Here's how the part is built. I have some questions about the finished solid (model axes, mm). Coordinates: 2 decimals unless noted, no trailing zeros. Order: outer loops, then holes, each group sorted by start corner. A loop starts at its lowest first (then second) coordinate and runs counter-clockwise, first axis right, second up. Notation, with made-up numbers: (74, 65) - (87, 65) arc R23 ccw to (87, 98) - close; hole circle Ø4 at (22, 48.5). An arc over 180 degrees is marked (long way). Answer as CSV lines item,"result". Start each with the question number.
Item 1: Imagine slicing it at A-A on y = 546. List the corners of the cut face in (x, z) for me, and give its area (3 significant figures).
Item 2: Imagine slicing it at B-B on y = 535. List the corners of the cut face in (x, z) for me, and give its area (3 significant figures).
Item 3: I need wall thicknesses on line 1 (Y direction, x = -537, z = -80.75); line 2 (X direction, y = 515.5, z = -81); line 3 (X direction, y = 514, z = -82.75). Which ranges of each line are inside material? Lowest first, please.
Item 4: Imagine slicing it at C-C on x = -570. Count the separate pieces of the cut face and the enclosed holes in it, and give its area (3 significant figures).
Item 5: We'd pull the mould along Y, two halves only. Please class faces 1 (the face through (-650.1, 527.3, -81)), 2 (the face through (-530.587, 524, -81)), 3 (the face through (-549, 531.139, -82)), 4 (the face through (-566, 513.156, -82)): pulls with the +Y half, pulls with the -Y half, needs draft (parallel to the pull), parting line crosses it, or undercut.
Item 6: I'm going to push flat-ended pins straight in: pin 1 (3 mm diameter, centred on x = -634, z = -81, fed in from -Y); pin 2 (1.4 mm diameter, centred on y = 511.5, z = -82, fed in from -X); pin 3 (1.3 mm diameter, centred on y = 499.5, z = -79, fed in from -X); pin 4 (4 mm diameter, centred on x = -569.5, y = 534.5, fed in from -Z). Where does each tip first touch, or does it pass through?
from build123d import *

# Parameters (mm, degrees)
SKETCH2_W                                       = 12.7
SKETCH2_H                                       = 6.604
SKETCH2_W_2                                     = 16.7132
SKETCH2_H_2                                     = 16.7132
BOSS_EXTRUDE1_DEPTH                             = 6.35
CBORE_FOR_6_PAN_HEAD_MACHINE_SCREW1_D           = 4.3053
CBORE_FOR_6_PAN_HEAD_MACHINE_SCREW1_CBORE_D     = 7.54126
CBORE_FOR_6_PAN_HEAD_MACHINE_SCREW1_CBORE_DEPTH = 2.4638
F_6_THREADED_INSERT_TAPERED_HOLE_AT_2_COUNT     = 2
F_6_THREADED_INSERT_TAPERED_HOLE_AT_2_PITCH     = 71.875418055
F_6_THREADED_INSERT_TAPERED_HOLE_AT_3_COUNT     = 2
F_6_THREADED_INSERT_TAPERED_HOLE_AT_3_PITCH     = 82.118347554
SKETCH7_W                                       = 16.7132
SKETCH7_H                                       = 16.7132
CUT_EXTRUDE1_DEPTH                              = 7.35
SKETCH8_W                                       = 14.224
SKETCH8_H                                       = 8.128
SKETCH8_W_2                                     = 18.2372
SKETCH8_H_2                                     = 18.2372
CUT_EXTRUDE2_DEPTH                              = 4.7625
FILLET1_R                                       = 1.5875
F_4_CLEARANCE_HOLE1_D                           = 3.4544
F_4_CLEARANCE_HOLE2_D                           = 3.4544
F_4_CLEARANCE_HOLE2_DEPTH                       = 1.5875
F_6_CLEARANCE_HOLE1_D                           = 4.3053


with BuildPart() as part:
    # Sketch2 → Boss-Extrude1 (new body)
    with BuildSketch(Plane.XY.offset(-77.851)):
        with BuildLine():
            Line((-530.586747576, 481.6475), (-530.586747576, 566.172689586))
            ThreePointArc((-530.586747576, 566.172689586), (-534.634798168, 572.345868951), (-541.909921986, 571.093898298))
            Line((-541.909921986, 571.093898298), (-585.196747576, 530.70125))
            Line((-585.196747576, 530.70125), (-644.251747576, 530.70125))
            ThreePointArc((-644.251747576, 530.70125), (-650.176036104, 527.165428624), (-649.876219443, 520.272726881))
            ThreePointArc((-649.876219443, 520.272726881), (-648.110778149, 517.987132771), (-646.019069209, 515.995782195))
            ThreePointArc((-646.019069209, 515.995782195), (-600.796684082, 490.491166469), (-549.636747576, 481.6475))
            Line((-549.636747576, 481.6475), (-530.586747576, 481.6475))
        make_face()
        with Locations((-566.019747576, 499.237)):
            Rectangle(SKETCH2_W, SKETCH2_H, mode=Mode.SUBTRACT)
        with Locations((-566.019747576, 508.2286)):
            Rectangle(SKETCH2_W, SKETCH2_H, mode=Mode.SUBTRACT)
        with Locations((-548.874747576, 499.237)):
            Rectangle(SKETCH2_W, SKETCH2_H, mode=Mode.SUBTRACT)
        with Locations((-548.874747576, 508.2286)):
            Rectangle(SKETCH2_W, SKETCH2_H, mode=Mode.SUBTRACT)
        with Locations((-548.874747576, 517.2202)):
            Rectangle(SKETCH2_W, SKETCH2_H, mode=Mode.SUBTRACT)
        with Locations((-566.019747576, 517.2202)):
            Rectangle(SKETCH2_W, SKETCH2_H, mode=Mode.SUBTRACT)
        with Locations((-566.019747576, 526.2118)):
            Rectangle(SKETCH2_W, SKETCH2_H, mode=Mode.SUBTRACT)
        with Locations((-548.874747576, 526.2118)):
            Rectangle(SKETCH2_W, SKETCH2_H, mode=Mode.SUBTRACT)
        with Locations((-548.874747576, 535.2034)):
            Rectangle(SKETCH2_W, SKETCH2_H, mode=Mode.SUBTRACT)
        with Locations((-566.019747576, 535.2034)):
            Rectangle(SKETCH2_W, SKETCH2_H, mode=Mode.SUBTRACT)
        with Locations((-548.874747576, 544.195)):
            Rectangle(SKETCH2_W, SKETCH2_H, mode=Mode.SUBTRACT)
        with Locations((-586.974747576, 512.7244)):
            Rectangle(SKETCH2_W_2, SKETCH2_H_2, mode=Mode.SUBTRACT)
    extrude(amount=-BOSS_EXTRUDE1_DEPTH)

    # CBORE for #6 Pan Head Machine Screw1 (through all)
    with Locations(Plane.XY.offset(-77.851)):
        with Locations((-537.317747576, 489.9025), (-537.317747576, 566.172689586), (-644.251747576, 523.97025)):
            CounterBoreHole(CBORE_FOR_6_PAN_HEAD_MACHINE_SCREW1_D / 2, CBORE_FOR_6_PAN_HEAD_MACHINE_SCREW1_CBORE_D / 2, CBORE_FOR_6_PAN_HEAD_MACHINE_SCREW1_CBORE_DEPTH)

    # Sketch5 → #6 Threaded Insert Tapered Hole (revolve, cut)
    with BuildSketch(Plane(origin=(-558.526747576, 487.9975, -77.851), x_dir=(0, -1, 0), z_dir=(1, 0, 0))):
        Polygon((0, 0), (0, 3.81), (2.5273, 3.81), (2.6543, 0), align=None)
    f_6_threaded_insert_tapered_hole = revolve(axis=Axis((-558.526747576, 487.9975, -187.851), (0, 0, 1)), mode=Mode.SUBTRACT)

    # #6 Threaded Insert Tapered Hole at 2: #6 Threaded Insert Tapered Hole ×2
    with Locations(*[Vector(0.159025162, 0.98727453, 0) * (i * F_6_THREADED_INSERT_TAPERED_HOLE_AT_2_PITCH) for i in range(1, F_6_THREADED_INSERT_TAPERED_HOLE_AT_2_COUNT)]):
        add(f_6_threaded_insert_tapered_hole, mode=Mode.SUBTRACT)

    # #6 Threaded Insert Tapered Hole at 3: #6 Threaded Insert Tapered Hole ×2
    with Locations(*[Vector(-0.889265337, 0.457391693, 0) * (i * F_6_THREADED_INSERT_TAPERED_HOLE_AT_3_PITCH) for i in range(1, F_6_THREADED_INSERT_TAPERED_HOLE_AT_3_COUNT)]):
        add(f_6_threaded_insert_tapered_hole, mode=Mode.SUBTRACT)

    # Sketch7 → Cut-Extrude1 (cut, through all)
    with BuildSketch(Plane.XY.offset(-77.851)):
        with Locations((-610.948497092, 512.7244)):
            Rectangle(SKETCH7_W, SKETCH7_H)
    extrude(amount=-CUT_EXTRUDE1_DEPTH, mode=Mode.SUBTRACT)

    # Sketch8 → Cut-Extrude2 (cut)
    with BuildSketch(Plane(origin=(0, 0, -84.201), x_dir=(-1, 0, 0), z_dir=(0, 0, -1))):
        with Locations((548.874747576, 544.195)):
            Rectangle(SKETCH8_W, SKETCH8_H)
        with Locations((548.874747576, 535.2034)):
            Rectangle(SKETCH8_W, SKETCH8_H)
        with Locations((548.874747576, 526.2118)):
            Rectangle(SKETCH8_W, SKETCH8_H)
        with Locations((548.874747576, 517.2202)):
            Rectangle(SKETCH8_W, SKETCH8_H)
        with Locations((548.874747576, 508.2286)):
            Rectangle(SKETCH8_W, SKETCH8_H)
        with Locations((548.874747576, 499.237)):
            Rectangle(SKETCH8_W, SKETCH8_H)
        with Locations((566.019747576, 535.2034)):
            Rectangle(SKETCH8_W, SKETCH8_H)
        with Locations((566.019747576, 526.2118)):
            Rectangle(SKETCH8_W, SKETCH8_H)
        with Locations((566.019747576, 517.2202)):
            Rectangle(SKETCH8_W, SKETCH8_H)
        with Locations((566.019747576, 508.2286)):
            Rectangle(SKETCH8_W, SKETCH8_H)
        with Locations((566.019747576, 499.237)):
            Rectangle(SKETCH8_W, SKETCH8_H)
        with Locations((586.974747576, 512.7244)):
            Rectangle(SKETCH8_W_2, SKETCH8_H_2)
        with Locations((610.948497092, 512.7244)):
            Rectangle(SKETCH8_W_2, SKETCH8_H_2)
    extrude(amount=-CUT_EXTRUDE2_DEPTH, mode=Mode.SUBTRACT)

    # Fillet1
    fillet1_edges = [part.edges().sort_by_distance(p)[0] for p in [
        (-585.196747576, 530.70125, -81.026),
        (-530.586747576, 481.6475, -81.026),
    ]]
    fillet(fillet1_edges, radius=FILLET1_R)

    # #4 Clearance Hole1 (through all)
    with Locations(Plane.XY.offset(-77.851)):
        with Locations((-537.317747576, 502.637594793), (-537.317747576, 553.437594793)):
            Hole(F_4_CLEARANCE_HOLE1_D / 2)

    # Sketch11 → Hole2 (revolve, cut)
    with BuildSketch(Plane(origin=(-642.655514401, 517.992624646, -84.201), x_dir=(0, 1, 0), z_dir=(1, 0, 0))):
        Polygon((0, 0), (0, 3.429), (1.9431, 3.429), (2.0701, 0), align=None)
    revolve(axis=Axis((-642.655514401, 517.992624646, 25.799), (0, 0, -1)), mode=Mode.SUBTRACT)

    # #4 Clearance Hole2
    with Locations(Plane(origin=(0, 0, -80.772), x_dir=(-1, 0, 0), z_dir=(0, 0, -1))):
        with Locations((642.655514401, 517.992624646)):
            Hole(F_4_CLEARANCE_HOLE2_D / 2, depth=F_4_CLEARANCE_HOLE2_DEPTH)

    # #6 Clearance Hole1 (through all)
    with Locations(Plane.XY.offset(-81.661)):
        with Locations((-558.526747576, 487.9975), (-631.551747576, 525.55775), (-547.096747576, 558.958269588)):
            Hole(F_6_CLEARANCE_HOLE1_D / 2)


solid = part.part
Responses:
1,outline,"(-568.8, -84.2) - (-555.99, -84.2) - (-555.99, -79.44) - (-555.22, -79.44) - (-555.22, -77.85) - (-568.8, -77.85) - close; (-542.52, -79.44) - (-541.76, -79.44) - (-541.76, -84.2) - (-530.59, -84.2) - (-530.59, -77.85) - (-542.52, -77.85) - close"
1,area,"155 mm^2"
2,outline,"(-580.59, -84.2) - (-573.13, -84.2) - (-573.13, -79.44) - (-572.37, -79.44) - (-572.37, -77.85) - (-580.59, -77.85) - close; (-559.67, -79.44) - (-558.91, -79.44) - (-558.91, -84.2) - (-555.99, -84.2) - (-555.99, -79.44) - (-555.22, -79.44) - (-555.22, -77.85) - (-559.67, -77.85) - close; (-542.52, -79.44) - (-541.76, -79.44) - (-541.76, -84.2) - (-530.59, -84.2) - (-530.59, -77.85) - (-542.52, -77.85) - close"
2,area,"142 mm^2"
3,line 1,"y = 481.65 to 487.77, 492.03 to 500.94, 504.34 to 551.74, 555.14 to 564.04, 568.3 to 572.9"
3,line 2,"x = -645.41 to -620.07, -601.83 to -596.09, -577.86 to -573.13, -558.91 to -555.99, -541.76 to -530.59"
3,line 3,"x = -643.52 to -620.07, -601.83 to -596.09, -577.86 to -573.13, -558.91 to -555.99, -541.76 to -530.59"
4,separate pieces,"6"
4,enclosed holes,"0"
4,area,"147 mm^2"
5,face 1,"parting line crosses it"
5,face 2,"needs draft"
5,face 3,"undercut"
5,face 4,"undercut"
6,pin 1,"stops at y = 506.14"
6,pin 2,"stops at x = -641.17"
6,pin 3,"stops at x = -622.42"
6,pin 4,"passes through"
